from build123d import *

# Parameters (mm, degrees)
F1_DEPTH     = 41
F3_DEPTH     = 38.5
F5_T1_DEPTH  = 38.46
F5_T3_DEPTH  = 179.905
F5_T5_DEPTH  = 106.405
F5_T7_DEPTH  = 47.35
F5_T9_DEPTH  = 42.905
F5_T11_DEPTH = 78.175
F5_T13_DEPTH = 41.175
F5_T15_DEPTH = 67.175
F5_T17_DEPTH = 67.175
F5_T19_DEPTH = 40.905
F5_T21_DEPTH = 101.96
F5_S25_W     = 1.27
F5_S25_H     = 1.27
F5_T26_DEPTH = 1.27
F5_S31_W     = 1.27
F5_S31_H     = 1.27
F5_T32_DEPTH = 1.27
F5_S37_W     = 1.27
F5_S37_H     = 1.27
F5_T38_DEPTH = 1.27
F5_T45_DEPTH = 81.35
F5_T49_DEPTH = 44.35
F5_T56_DEPTH = 70.35
F5_T60_DEPTH = 70.35


# Not quite as in the source:
# - a fillet or chamfer that OpenCascade refuses, or shapes differently, is made with other operations: its cross-section is extruded or revolved along the edge and cut away or added
# - a feature of the source that left no trace in its solid (it failed there, or was rolled back) is left out


with BuildPart() as f1:
    # F0 (on Top) → F1 (new body)
    with BuildSketch(Plane.XY):
        Polygon((0, 102.9857128358), (0, 0), (0, -75.0142871642), (2.5, -75.0142871642), (2.5, -0.0142871642), (40.5, -0.0142871642), (40.5, 63.9857128358), (104.5, 63.9857128358), (104.5, 102.9857128358), align=None)
    extrude(amount=F1_DEPTH)

    # F2 (on face) → F3 (cut)
    with BuildSketch(Plane.XY.offset(41)):
        Polygon((2.5, 100.4857128358), (2.5, -0.0142871642), (40.5, -0.0142871642), (40.5, 63.9857128358), (104.5, 63.9857128358), (104.5, 100.4857128358), align=None)
    extrude(amount=-F3_DEPTH, mode=Mode.SUBTRACT)

    # F5: fillet of radius 1.27 on 12 edges, made by hand

    # F5_s2 → F5_t1 (cut)
    with BuildSketch(Plane.XY.offset(1.27)):
        with BuildLine():
            ThreePointArc((0, 101.7157128358), (0.3719743879, 102.6137384479), (1.27, 102.9857128358))
            Line((1.27, 102.9857128358), (0, 102.9857128358))
            Line((0, 102.9857128358), (0, 101.7157128358))
        make_face()
    extrude(amount=F5_T1_DEPTH, mode=Mode.SUBTRACT)

    # F5_s4 → F5_t3 (cut)
    with BuildSketch(Plane.XZ.offset(-101.7157128358)):
        with BuildLine():
            ThreePointArc((0, 39.73), (0.3719743879, 40.6280256121), (1.27, 41))
            Line((1.27, 41), (0, 41))
            Line((0, 41), (0, 39.73))
        make_face()
        with BuildLine():
            ThreePointArc((0, 1.27), (0.3719743879, 0.3719743879), (1.27, 0))
            Line((1.27, 0), (0, 0))
            Line((0, 0), (0, 1.27))
        make_face()
    extrude(amount=F5_T3_DEPTH, mode=Mode.SUBTRACT)

    # F5_s6 → F5_t5 (cut)
    with BuildSketch(Plane.YZ.offset(1.27)):
        with BuildLine():
            ThreePointArc((101.7157128358, 41), (102.6137384479, 40.6280256121), (102.9857128358, 39.73))
            Line((102.9857128358, 39.73), (102.9857128358, 41))
            Line((102.9857128358, 41), (101.7157128358, 41))
        make_face()
    extrude(amount=F5_T5_DEPTH, mode=Mode.SUBTRACT)

    # F5_s8 → F5_t7 (cut)
    with BuildSketch(Plane.XY.offset(-3.175)):
        with BuildLine():
            ThreePointArc((0, -73.7442871642), (0.3719743879, -74.6423127763), (1.27, -75.0142871642))
            Line((1.27, -75.0142871642), (0, -75.0142871642))
            Line((0, -75.0142871642), (0, -73.7442871642))
        make_face()
    extrude(amount=F5_T7_DEPTH, mode=Mode.SUBTRACT)

    # F5_s10 → F5_t9 (cut)
    with BuildSketch(Plane.XY.offset(1.27)):
        with BuildLine():
            ThreePointArc((104.5, 101.7157128358), (104.1280256121, 102.6137384479), (103.23, 102.9857128358))
            Line((103.23, 102.9857128358), (104.5, 102.9857128358))
            Line((104.5, 102.9857128358), (104.5, 101.7157128358))
        make_face()
    extrude(amount=F5_T9_DEPTH, mode=Mode.SUBTRACT)

    # F5_s12 → F5_t11 (cut)
    with BuildSketch(Plane.XZ.offset(0.0142871642)):
        with BuildLine():
            ThreePointArc((1.23, 0), (2.1280256121, 0.3719743879), (2.5, 1.27))
            Line((2.5, 1.27), (2.5, 0))
            Line((2.5, 0), (1.23, 0))
        make_face()
    extrude(amount=F5_T11_DEPTH, mode=Mode.SUBTRACT)

    # F5_s14 → F5_t13 (cut)
    with BuildSketch(Plane.YZ.offset(2.5)):
        with BuildLine():
            ThreePointArc((1.2557128358, 0), (0.3576872237, 0.3719743879), (-0.0142871642, 1.27))
            Line((-0.0142871642, 1.27), (-0.0142871642, 0))
            Line((-0.0142871642, 0), (1.2557128358, 0))
        make_face()
    extrude(amount=F5_T13_DEPTH, mode=Mode.SUBTRACT)

    # F5_s16 → F5_t15 (cut)
    with BuildSketch(Plane.XZ.offset(-63.9857128358)):
        with BuildLine():
            ThreePointArc((39.23, 0), (40.1280256121, 0.3719743879), (40.5, 1.27))
            Line((40.5, 1.27), (40.5, 0))
            Line((40.5, 0), (39.23, 0))
        make_face()
    extrude(amount=F5_T15_DEPTH, mode=Mode.SUBTRACT)

    # F5_s18 → F5_t17 (cut)
    with BuildSketch(Plane.YZ.offset(40.5)):
        with BuildLine():
            ThreePointArc((65.2557128358, 0), (64.3576872237, 0.3719743879), (63.9857128358, 1.27))
            Line((63.9857128358, 1.27), (63.9857128358, 0))
            Line((63.9857128358, 0), (65.2557128358, 0))
        make_face()
    extrude(amount=F5_T17_DEPTH, mode=Mode.SUBTRACT)

    # F5_s20 → F5_t19 (cut)
    with BuildSketch(Plane.XZ.offset(-101.7157128358)):
        with BuildLine():
            ThreePointArc((103.23, 0), (104.1280256121, 0.3719743879), (104.5, 1.27))
            Line((104.5, 1.27), (104.5, 0))
            Line((104.5, 0), (103.23, 0))
        make_face()
    extrude(amount=F5_T19_DEPTH, mode=Mode.SUBTRACT)

    # F5_s22 → F5_t21 (cut)
    with BuildSketch(Plane.YZ.offset(1.27)):
        with BuildLine():
            ThreePointArc((101.7157128358, 0), (102.6137384479, 0.3719743879), (102.9857128358, 1.27))
            Line((102.9857128358, 1.27), (102.9857128358, 0))
            Line((102.9857128358, 0), (101.7157128358, 0))
        make_face()
    extrude(amount=F5_T21_DEPTH, mode=Mode.SUBTRACT)


with BuildPart() as f5_tool24:
    # F5_s25 → F5_t26 (new body)
    with BuildSketch(Plane.YZ.offset(1.27)):
        with Locations((102.3507128358, 0.635)):
            Rectangle(F5_S25_W, F5_S25_H)
    extrude(amount=-F5_T26_DEPTH)

    # F5_s27 → F5_t28 (revolve, cut)
    with BuildSketch(Plane(origin=(1.27, 101.7157128358, 1.27), x_dir=(0, -0.7071067812, 0.7071067812), z_dir=(0, -0.7071067812, -0.7071067812))):
        with BuildLine():
            ThreePointArc((0, -1.27), (1.27, 0), (0, 1.27))
            Line((0, 1.27), (0, -1.27))
        make_face()
    revolve(axis=Axis((1.27, 101.7157128358, 1.27), (-1, 0, 0)), mode=Mode.SUBTRACT)


with BuildPart() as f1_1:
    add(f1.part)

    # F5_t23: cut F5_tool24
    add(f5_tool24.part, mode=Mode.SUBTRACT)


with BuildPart() as f5_tool30:
    # F5_s31 → F5_t32 (new body)
    with BuildSketch(Plane.YZ.offset(1.27)):
        with Locations((102.3507128358, 40.365)):
            Rectangle(F5_S31_W, F5_S31_H)
    extrude(amount=-F5_T32_DEPTH)

    # F5_s33 → F5_t34 (revolve, cut)
    with BuildSketch(Plane(origin=(1.27, 101.7157128358, 39.73), x_dir=(0, -0.7071067812, -0.7071067812), z_dir=(0, 0.7071067812, -0.7071067812))):
        with BuildLine():
            ThreePointArc((0, -1.27), (1.27, 0), (0, 1.27))
            Line((0, 1.27), (0, -1.27))
        make_face()
    revolve(axis=Axis((1.27, 101.7157128358, 39.73), (-1, 0, 0)), mode=Mode.SUBTRACT)


with BuildPart() as f1_2:
    add(f1_1.part)

    # F5_t29: cut F5_tool30
    add(f5_tool30.part, mode=Mode.SUBTRACT)


with BuildPart() as f5_tool36:
    # F5_s37 → F5_t38 (new body)
    with BuildSketch(Plane.XY.offset(1.27)):
        with Locations((103.865, 102.3507128358)):
            Rectangle(F5_S37_W, F5_S37_H)
    extrude(amount=-F5_T38_DEPTH)

    # F5_s39 → F5_t40 (revolve, cut)
    with BuildSketch(Plane(origin=(103.23, 101.7157128358, 1.27), x_dir=(-0.7071067812, -0.7071067812, 0), z_dir=(0.7071067812, -0.7071067812, 0))):
        with BuildLine():
            ThreePointArc((0, -1.27), (1.27, 0), (0, 1.27))
            Line((0, 1.27), (0, -1.27))
        make_face()
    revolve(axis=Axis((103.23, 101.7157128358, 1.27), (0, 0, -1)), mode=Mode.SUBTRACT)


with BuildPart() as f1_3:
    add(f1_2.part)

    # F5_t35: cut F5_tool36
    add(f5_tool36.part, mode=Mode.SUBTRACT)


with BuildPart() as f5_tool43:
    # F5_s44 → F5_t45 (new body)
    with BuildSketch(Plane.XZ.offset(78.1892871642)):
        with BuildLine():
            ThreePointArc((1.23, 0), (2.1280256121, 0.3719743879), (2.5, 1.27))
            Line((2.5, 1.27), (2.5, 0))
            Line((2.5, 0), (1.23, 0))
        make_face()
    extrude(amount=-F5_T45_DEPTH)

    split(bisect_by=Plane.XZ.offset(0.0142871642), keep=Keep.BOTTOM)


with BuildPart() as f5_tool47:
    # F5_s48 → F5_t49 (new body)
    with BuildSketch(Plane.YZ.offset(-0.675)):
        with BuildLine():
            ThreePointArc((1.2557128358, 0), (0.3576872237, 0.3719743879), (-0.0142871642, 1.27))
            Line((-0.0142871642, 1.27), (-0.0142871642, 0))
            Line((-0.0142871642, 0), (1.2557128358, 0))
        make_face()
    extrude(amount=F5_T49_DEPTH)

    split(bisect_by=Plane.YZ.offset(2.5), keep=Keep.BOTTOM)


with BuildPart() as f5_tool43_1:
    add(f5_tool43.part)

    # F5_t51: intersect F5_tool47
    add(f5_tool47.part, mode=Mode.INTERSECT)


with BuildPart() as f1_4:
    add(f1_3.part)

    # F5_t41: cut F5_tool43
    add(f5_tool43_1.part, mode=Mode.SUBTRACT)


with BuildPart() as f5_tool54:
    # F5_s55 → F5_t56 (new body)
    with BuildSketch(Plane.XZ.offset(3.1892871642)):
        with BuildLine():
            ThreePointArc((39.23, 0), (40.1280256121, 0.3719743879), (40.5, 1.27))
            Line((40.5, 1.27), (40.5, 0))
            Line((40.5, 0), (39.23, 0))
        make_face()
    extrude(amount=-F5_T56_DEPTH)

    split(bisect_by=Plane.XZ.offset(-63.9857128358), keep=Keep.BOTTOM)


with BuildPart() as f5_tool58:
    # F5_s59 → F5_t60 (new body)
    with BuildSketch(Plane.YZ.offset(37.325)):
        with BuildLine():
            ThreePointArc((65.2557128358, 0), (64.3576872237, 0.3719743879), (63.9857128358, 1.27))
            Line((63.9857128358, 1.27), (63.9857128358, 0))
            Line((63.9857128358, 0), (65.2557128358, 0))
        make_face()
    extrude(amount=F5_T60_DEPTH)

    split(bisect_by=Plane.YZ.offset(40.5), keep=Keep.BOTTOM)


with BuildPart() as f5_tool54_1:
    add(f5_tool54.part)

    # F5_t62: intersect F5_tool58
    add(f5_tool58.part, mode=Mode.INTERSECT)


with BuildPart() as f1_5:
    add(f1_4.part)

    # F5_t52: cut F5_tool54
    add(f5_tool54_1.part, mode=Mode.SUBTRACT)


solid = f1_5.part
The listing builds one solid part. Answer for the finished solid, in the listing's coordinates (mm). A direction names the side the tool comes from. Coordinates: 2 decimals unless noted, no trailing zeros. Loops run counter-clockwise (first coordinate to the right, second up) from the corner with the lowest first, then second, coordinate; pieces in that order, holes last. Notation, with made-up numbers: (9.25, 36.5) -> (29.25, 36.5) arc R10 ccw to (29.25, 54.5) -> close; hole circle Ø10 at (60.25, -27.75). An arc over 180 degrees is marked (long way). Answer in a Markdown table with one row per item. Add a question column.
1. Flat-ended cylindrical pins translate along their axes: P1, Ø20, axis at y = -17.5, z = 30, coming from the +X side; P2, Ø19, axis at x = 53, z = 15, coming from the -Y side; P3, Ø1.4, axis at y = 16.5, z = 2, coming from the +X side. Find the tip coordinate at first contact, or state that the pin passes through.
2. Consider line 1 (X direction, y = -5, z = 4.5); line 2 (Y direction, x = 18.5, z = 35). Determine where each line is inside the solid, lowest interval first. Write a range as [from, to].
3. The part is cut by section B-B, the plane z = 31. Write down the section's boundary in (x, y), then the cut area to 3 significant figures.
4. The part is cut by section C-C, the plane y = -33.5. Write down the section's boundary in (x, z), then the cut area to 3 significant figures.
5. For faces 1 (the flat face through (0, 15, 20)), 2 (the flat face through (41, 73, 2.5)), determine the directions among +Z, -Z, +X, -X, +Y, -Y from which every point of the face is accessible in a straight line to the end or side of a thin tool.
6. The part is cut by section A-A, the plane x = 61.5. Write down the section's boundary in (y, z).
Answer below:
| question | item | result |
|---|---|---|
| 1 | P1 | x = 2.5 |
| 1 | P2 | y = 100.49 |
| 1 | P3 | x = 40.5 |
| 2 | line 1 | [0, 2.5] |
| 2 | line 2 | [100.49, 102.99] |
| 3 | outline | (0, -73.74) arc R1.27 ccw to (1.27, -75.01) -> (2.5, -75.01) -> (2.5, 100.49) -> (104.5, 100.49) -> (104.5, 101.72) arc R1.27 ccw to (103.23, 102.99) -> (1.27, 102.99) arc R1.27 ccw to (0, 101.72) -> close |
| 3 | area | 699 mm2 |
| 4 | outline | (0, 1.27) arc R1.27 ccw to (1.25, 0) arc R1.27 ccw to (2.5, 1.27) -> (2.5, 41) -> (1.27, 41) arc R1.27 ccw to (0, 39.73) -> close |
| 4 | area | 101 mm2 |
| 5 | face 1 | +Z, -Z, -X, +Y, -Y |
| 5 | face 2 | +Z, +X, -Y |
| 6 | outline | (63.99, 1.27) arc R1.27 ccw to (65.26, 0) -> (101.72, 0) arc R1.27 ccw to (102.99, 1.27) -> (102.99, 39.73) arc R1.27 ccw to (101.72, 41) -> (100.49, 41) -> (100.49, 2.5) -> (63.99, 2.5) -> close |
